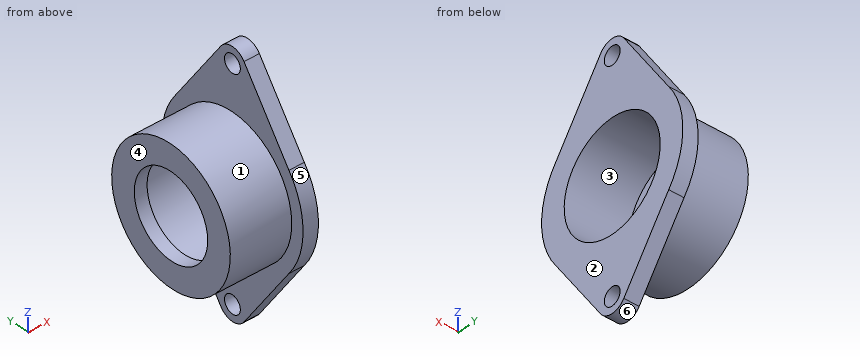
```python
from build123d import *

# Parameters (mm, degrees)
BOSS_EXTRUDE1_START     = -12
SKETCH2_R               = 52.5
BOSS_EXTRUDE1_DEPTH     = 12
CUT_EXTRUDE1_DEPTH      = 158.743730759
CUT_EXTRUDE1_DEPTH_BACK = 158.743730759
SKETCH3_R               = 7


with BuildPart() as part:
    # Sketch1 → Revolve1 (revolve)
    with BuildSketch(Plane.XY, mode=Mode.PRIVATE) as revolve1_sk:
        Polygon((-43.504823151, -1.221864952), (6.495176849, -1.221864952), (6.495176849, 8.778135048), (-53.504823151, 8.778135048), (-53.504823151, -11.221864952), (-43.504823151, -11.221864952), align=None)
    revolve(revolve1_sk.sketch.rotate(Axis((-50.064308682, -43.721864952, 0), (1, 0, 0)), 90), axis=Axis((-50.064308682, -43.721864952, 0), (1, 0, 0)))

    # Sketch2 → Boss-Extrude1 (add)
    with BuildSketch(Plane(origin=(6.495176849, 0, 0), x_dir=(0, 0, -1), z_dir=(1, 0, 0)).offset(BOSS_EXTRUDE1_START)):
        with BuildLine():
            Line((-37.500000001, -93.721864951), (-94.637131817, -53.983996769))
            ThreePointArc((-94.637131817, -53.983996769), (-100, -43.721864952), (-94.637131817, -33.459733135))
            Line((-94.637131817, -33.459733135), (-37.500000001, 6.278135048))
            ThreePointArc((-37.500000001, 6.278135048), (0, 18.778135048), (37.500000001, 6.278135048))
            Line((37.500000001, 6.278135048), (94.637131817, -33.459733135))
            ThreePointArc((94.637131817, -33.459733135), (100, -43.721864952), (94.637131817, -53.983996769))
            Line((94.637131817, -53.983996769), (37.500000001, -93.721864951))
            ThreePointArc((37.500000001, -93.721864951), (0, -106.221864952), (-37.500000001, -93.721864951))
        make_face()
        with Locations(Location((0, -43.721864952, 0), (0, 0, 180))):
            Circle(SKETCH2_R, mode=Mode.SUBTRACT)
    extrude(amount=BOSS_EXTRUDE1_DEPTH)

    # Sketch3 → Cut-Extrude1 (cut, two sides: drawn at the far end of the back side and taken through both)
    with BuildSketch(Plane(origin=(6.495176849, 0, 0), x_dir=(0, 0, -1), z_dir=(1, 0, 0)).offset(-CUT_EXTRUDE1_DEPTH_BACK)):
        with Locations((87.5, -43.721864952)):
            Circle(SKETCH3_R)
        with Locations((-87.5, -43.721864952)):
            Circle(SKETCH3_R)
    extrude(amount=CUT_EXTRUDE1_DEPTH + CUT_EXTRUDE1_DEPTH_BACK, mode=Mode.SUBTRACT)


solid = part.part
```
Verification items for the finished model (mm, model axes). Face numbers are marked on the shaded views. A direction names the side the tool comes from. Give positions to 0.01 mm unless a question says otherwise; leave off trailing zeros. Loops run counter-clockwise (first coordinate to the right, second up) from the corner with the lowest first, then second, coordinate; pieces in that order, holes last.
1. Thickness scan on line 1 (Y direction, x = -10, z = 0); line 2 (X direction, y = -71, z = 47); line 3 (X direction, y = -47.5, z = 34). Record the ranges inside material, lowest first.
2. Section check B-B, the plane y = -70.5. Enter the section's corners in (x, z).
3. Section check D-D, the plane x = -29.5. Enter the section's corners in (y, z).
4. Go/stop test with flat-tipped pins: pin 1 Ø6 at (x, y) = (-27.5, -25.5) entering from -Z; pin 2 Ø8 at (x, z) = (-38.5, -38.5) entering from +Y; pin 3 Ø12 at (x, z) = (-2, 15) entering from -Y; pin 4 Ø4 at (x, z) = (-47, 55) entering from -Y. Record where each tip stops, or that it passes through.
5. Section check C-C, the plane y = -6. Enter the section's corners in (x, z).
6. Mould release check, pull along Y, two halves, no side actions. Record for the marked faces 3, 4, 5 and 6: released by +Y, released by -Y, zero draft, split by the parting line, or undercut.
7. Set-up check for the marked faces 1 and 2: record each of +Z, -Z, +X, -X, +Y, -Y from which the full face is reachable in a straight line by a thin tool's end or side.
8. Section check A-A, the plane z = 0. Enter the section's corners in (x, y).
Geometry says:
1. line 1: y = -96.22 to -86.22, -1.22 to 8.78
1. line 2: x = -5.5 to 6.5
1. line 3: x = -53.5 to -43.5
2. outline: (-53.5, -45.16) - (-5.5, -45.16) - (-5.5, -70.89) - (6.5, -70.89) - (6.5, -33) - (-43.5, -33) - (-43.5, -18.42) - (-53.5, -18.42) - close; (-53.5, 18.42) - (-43.5, 18.42) - (-43.5, 33) - (6.5, 33) - (6.5, 70.89) - (-5.5, 70.89) - (-5.5, 45.16) - (-53.5, 45.16) - close
3. outline: circle Ø105 at (-43.72, 0); hole circle Ø85 at (-43.72, 0)
4. pin 1: stops at z = -50.24
4. pin 2: stops at y = -4.15
4. pin 3: stops at y = -105.57
4. pin 4: passes through
5. outline: (-53.5, -36.51) - (-5.5, -36.51) - (-5.5, -55.15) - (6.5, -55.15) - (6.5, -19.58) - (-43.5, -19.58) - (-43.5, 19.58) - (6.5, 19.58) - (6.5, 55.15) - (-5.5, 55.15) - (-5.5, 36.51) - (-53.5, 36.51) - close
6. face 3: undercut
6. face 4: zero draft
6. face 5: released by -Y
6. face 6: split by the parting line
7. face 1: -X
7. face 2: +Z, -Z, +X, +Y, -Y
8. outline: (-53.5, -96.22) - (-5.5, -96.22) - (-5.5, -106.22) - (6.5, -106.22) - (6.5, -86.22) - (-43.5, -86.22) - (-43.5, -76.22) - (-53.5, -76.22) - close; (-53.5, -11.22) - (-43.5, -11.22) - (-43.5, -1.22) - (6.5, -1.22) - (6.5, 18.78) - (-5.5, 18.78) - (-5.5, 8.78) - (-53.5, 8.78) - close
